Could you check a few things on this model? Use its own coordinates, in mm. Coordinates: 2 decimals unless noted, no trailing zeros. Put each result on its own line as item: value. Start each with the question number.
```python
from build123d import *

# Parameters (mm, degrees)
EXTRUDE_1_DEPTH = 400


with BuildPart() as part:
    # 草图1 → 凸台-拉伸1 (new body)
    with BuildSketch(Plane(origin=(0, 0, 0), x_dir=(1, 0, 0), z_dir=(0, 1, 0))):
        with BuildLine():
            Line((-3.476396103, 2.84), (-3.476396103, 0))
            Line((-3.476396103, 0), (-2.1, 0))
            ThreePointArc((-2.1, 0), (-1.48492424, 1.48492424), (0, 2.1))
            Line((0, 2.1), (0, 3.476396103))
            Line((0, 3.476396103), (-2.84, 3.476396103))
            Line((-2.84, 3.476396103), (-5.923603897, 6.56))
            Line((-5.923603897, 6.56), (-5.923603897, 8.2))
            Line((-5.923603897, 8.2), (-3.1, 8.2))
            Line((-3.1, 8.2), (-4.9, 10))
            Line((-4.9, 10), (-10, 10))
            Line((-10, 10), (-10, 4.9))
            Line((-10, 4.9), (-8.2, 3.1))
            Line((-8.2, 3.1), (-8.2, 5.923603897))
            Line((-8.2, 5.923603897), (-6.56, 5.923603897))
            Line((-6.56, 5.923603897), (-3.476396103, 2.84))
        make_face()
        with BuildLine():
            Line((-2.1, 0), (-3.476396103, 0))
            Line((-3.476396103, 0), (-3.476396103, -2.84))
            Line((-3.476396103, -2.84), (-6.56, -5.923603897))
            Line((-6.56, -5.923603897), (-8.2, -5.923603897))
            Line((-8.2, -5.923603897), (-8.2, -3.1))
            Line((-8.2, -3.1), (-10, -4.9))
            Line((-10, -4.9), (-10, -10))
            Line((-10, -10), (-4.9, -10))
            Line((-4.9, -10), (-3.1, -8.2))
            Line((-3.1, -8.2), (-5.923603897, -8.2))
            Line((-5.923603897, -8.2), (-5.923603897, -6.56))
            Line((-5.923603897, -6.56), (-2.84, -3.476396103))
            Line((-2.84, -3.476396103), (0, -3.476396103))
            Line((0, -3.476396103), (0, -2.1))
            ThreePointArc((0, -2.1), (-1.48492424, -1.48492424), (-2.1, 0))
        make_face()
        with BuildLine():
            ThreePointArc((2.1, 0), (1.48492424, -1.48492424), (0, -2.1))
            Line((0, -2.1), (0, -3.476396103))
            Line((0, -3.476396103), (2.84, -3.476396103))
            Line((2.84, -3.476396103), (5.923603897, -6.56))
            Line((5.923603897, -6.56), (5.923603897, -8.2))
            Line((5.923603897, -8.2), (3.1, -8.2))
            Line((3.1, -8.2), (4.9, -10))
            Line((4.9, -10), (15.1, -10))
            Line((15.1, -10), (16.9, -8.2))
            Line((16.9, -8.2), (14.076396103, -8.2))
            Line((14.076396103, -8.2), (14.076396103, -6.56))
            Line((14.076396103, -6.56), (17.16, -3.476396103))
            Line((17.16, -3.476396103), (20, -3.476396103))
            Line((20, -3.476396103), (20, -2.1))
            ThreePointArc((20, -2.1), (18.51507576, -1.48492424), (17.9, 0))
            Line((17.9, 0), (16.523603897, 0))
            Line((16.523603897, 0), (16.523603897, -2.84))
            Line((16.523603897, -2.84), (13.44, -5.923603897))
            Line((13.44, -5.923603897), (11.163603897, -8.2))
            Line((11.163603897, -8.2), (8.836396103, -8.2))
            Line((8.836396103, -8.2), (6.56, -5.923603897))
            Line((6.56, -5.923603897), (3.476396103, -2.84))
            Line((3.476396103, -2.84), (3.476396103, 0))
            Line((3.476396103, 0), (2.1, 0))
        make_face()
        with BuildLine():
            Line((0, 3.476396103), (0, 2.1))
            ThreePointArc((0, 2.1), (1.48492424, 1.48492424), (2.1, 0))
            Line((2.1, 0), (3.476396103, 0))
            Line((3.476396103, 0), (3.476396103, 2.84))
            Line((3.476396103, 2.84), (6.56, 5.923603897))
            Line((6.56, 5.923603897), (8.836396103, 8.2))
            Line((8.836396103, 8.2), (11.163603897, 8.2))
            Line((11.163603897, 8.2), (13.44, 5.923603897))
            Line((13.44, 5.923603897), (16.523603897, 2.84))
            Line((16.523603897, 2.84), (16.523603897, 0))
            Line((16.523603897, 0), (17.9, 0))
            ThreePointArc((17.9, 0), (18.51507576, 1.48492424), (20, 2.1))
            Line((20, 2.1), (20, 3.476396103))
            Line((20, 3.476396103), (17.16, 3.476396103))
            Line((17.16, 3.476396103), (14.076396103, 6.56))
            Line((14.076396103, 6.56), (14.076396103, 8.2))
            Line((14.076396103, 8.2), (16.9, 8.2))
            Line((16.9, 8.2), (15.1, 10))
            Line((15.1, 10), (4.9, 10))
            Line((4.9, 10), (3.1, 8.2))
            Line((3.1, 8.2), (5.923603897, 8.2))
            Line((5.923603897, 8.2), (5.923603897, 6.56))
            Line((5.923603897, 6.56), (2.84, 3.476396103))
            Line((2.84, 3.476396103), (0, 3.476396103))
        make_face()
        with BuildLine():
            Line((20, 3.476396103), (20, 2.1))
            ThreePointArc((20, 2.1), (21.48492424, 1.48492424), (22.1, 0))
            Line((22.1, 0), (23.476396103, 0))
            Line((23.476396103, 0), (23.476396103, 2.84))
            Line((23.476396103, 2.84), (26.56, 5.923603897))
            Line((26.56, 5.923603897), (28.836396103, 8.2))
            Line((28.836396103, 8.2), (31.163603897, 8.2))
            Line((31.163603897, 8.2), (33.44, 5.923603897))
            Line((33.44, 5.923603897), (36.523603897, 2.84))
            Line((36.523603897, 2.84), (36.523603897, 0))
            Line((36.523603897, 0), (37.9, 0))
            ThreePointArc((37.9, 0), (40, 2.1), (42.1, 0))
            Line((42.1, 0), (43.476396103, 0))
            Line((43.476396103, 0), (43.476396103, 2.84))
            Line((43.476396103, 2.84), (46.56, 5.923603897))
            Line((46.56, 5.923603897), (48.2, 5.923603897))
            Line((48.2, 5.923603897), (48.2, 3.1))
            Line((48.2, 3.1), (50, 4.9))
            Line((50, 4.9), (50, 10))
            Line((50, 10), (44.9, 10))
            Line((44.9, 10), (43.1, 8.2))
            Line((43.1, 8.2), (45.923603897, 8.2))
            Line((45.923603897, 8.2), (45.923603897, 6.56))
            Line((45.923603897, 6.56), (42.84, 3.476396103))
            Line((42.84, 3.476396103), (37.16, 3.476396103))
            Line((37.16, 3.476396103), (34.076396103, 6.56))
            Line((34.076396103, 6.56), (34.076396103, 8.2))
            Line((34.076396103, 8.2), (36.9, 8.2))
            Line((36.9, 8.2), (35.1, 10))
            Line((35.1, 10), (24.9, 10))
            Line((24.9, 10), (23.1, 8.2))
            Line((23.1, 8.2), (25.923603897, 8.2))
            Line((25.923603897, 8.2), (25.923603897, 6.56))
            Line((25.923603897, 6.56), (22.84, 3.476396103))
            Line((22.84, 3.476396103), (20, 3.476396103))
        make_face()
        with BuildLine():
            ThreePointArc((22.1, 0), (21.48492424, -1.48492424), (20, -2.1))
            Line((20, -2.1), (20, -3.476396103))
            Line((20, -3.476396103), (22.84, -3.476396103))
            Line((22.84, -3.476396103), (25.923603897, -6.56))
            Line((25.923603897, -6.56), (25.923603897, -8.2))
            Line((25.923603897, -8.2), (23.1, -8.2))
            Line((23.1, -8.2), (24.9, -10))
            Line((24.9, -10), (35.1, -10))
            Line((35.1, -10), (36.9, -8.2))
            Line((36.9, -8.2), (34.076396103, -8.2))
            Line((34.076396103, -8.2), (34.076396103, -6.56))
            Line((34.076396103, -6.56), (37.16, -3.476396103))
            Line((37.16, -3.476396103), (42.84, -3.476396103))
            Line((42.84, -3.476396103), (45.923603897, -6.56))
            Line((45.923603897, -6.56), (45.923603897, -8.2))
            Line((45.923603897, -8.2), (43.1, -8.2))
            Line((43.1, -8.2), (44.9, -10))
            Line((44.9, -10), (50, -10))
            Line((50, -10), (50, -4.9))
            Line((50, -4.9), (48.2, -3.1))
            Line((48.2, -3.1), (48.2, -5.923603897))
            Line((48.2, -5.923603897), (46.56, -5.923603897))
            Line((46.56, -5.923603897), (43.476396103, -2.84))
            Line((43.476396103, -2.84), (43.476396103, 0))
            Line((43.476396103, 0), (42.1, 0))
            ThreePointArc((42.1, 0), (40, -2.1), (37.9, 0))
            Line((37.9, 0), (36.523603897, 0))
            Line((36.523603897, 0), (36.523603897, -2.84))
            Line((36.523603897, -2.84), (33.44, -5.923603897))
            Line((33.44, -5.923603897), (31.163603897, -8.2))
            Line((31.163603897, -8.2), (28.836396103, -8.2))
            Line((28.836396103, -8.2), (26.56, -5.923603897))
            Line((26.56, -5.923603897), (23.476396103, -2.84))
            Line((23.476396103, -2.84), (23.476396103, 0))
            Line((23.476396103, 0), (22.1, 0))
        make_face()
    extrude(amount=EXTRUDE_1_DEPTH)


solid = part.part
```
(1) For pin 1 Ø1.7 at (x, y) = (19.5, 170.5) entering from +Z; pin 2 Ø3 at (y, z) = (241.5, -0.5) entering from +X; pin 3 Ø6 at (y, z) = (273.5, 1) entering from -X, each with a flat end and sliding along its axis, tell me the tip position at first contact or that it passes through.
(2) I want a section at A-A on y = 307.5. Count the separate pieces of the cut face and the enclosed holes in it, and give its area (3 significant figures).
(3) I need wall thicknesses on L1, parallel to X at y = 96, z = -2.25; L2, parallel to Z at x = 40, y = 97; L3, parallel to Z at x = 39.5, y = 67.5. Which ranges of each line are inside material? Lowest first, please. Write a range as [from, to].
Answer sheet:
1. pin 1: stops at z = 3.48
1. pin 2: stops at x = 43.48
1. pin 3: stops at x = -9.1
2. separate pieces: 1
2. enclosed holes: 5
2. area: 359 mm^2
3. L1: x = [-3.48, 3.48], [16.52, 23.48], [36.52, 43.48]
3. L2: z = [-3.48, -2.1], [2.1, 3.48]
3. L3: z = [-3.48, -2.04], [2.04, 3.48]
